Print and shaded views of the part. All mm, measured from the part's lowest x, y and z. A direction names the side the tool comes from. Coordinates: 2 decimals unless noted, no trailing zeros. Loops run counter-clockwise (first coordinate to the right, second up) from the corner with the lowest first, then second, coordinate; pieces in that order, holes last. Notation, with made-up numbers: M 44,30.5 L 59,30.5 A33 ccw 59,61.5 Z; hole C -24,62 d6. An arc over 180 degrees is marked long. Answer as a JSON object with one key per item and string values. Group by question number.
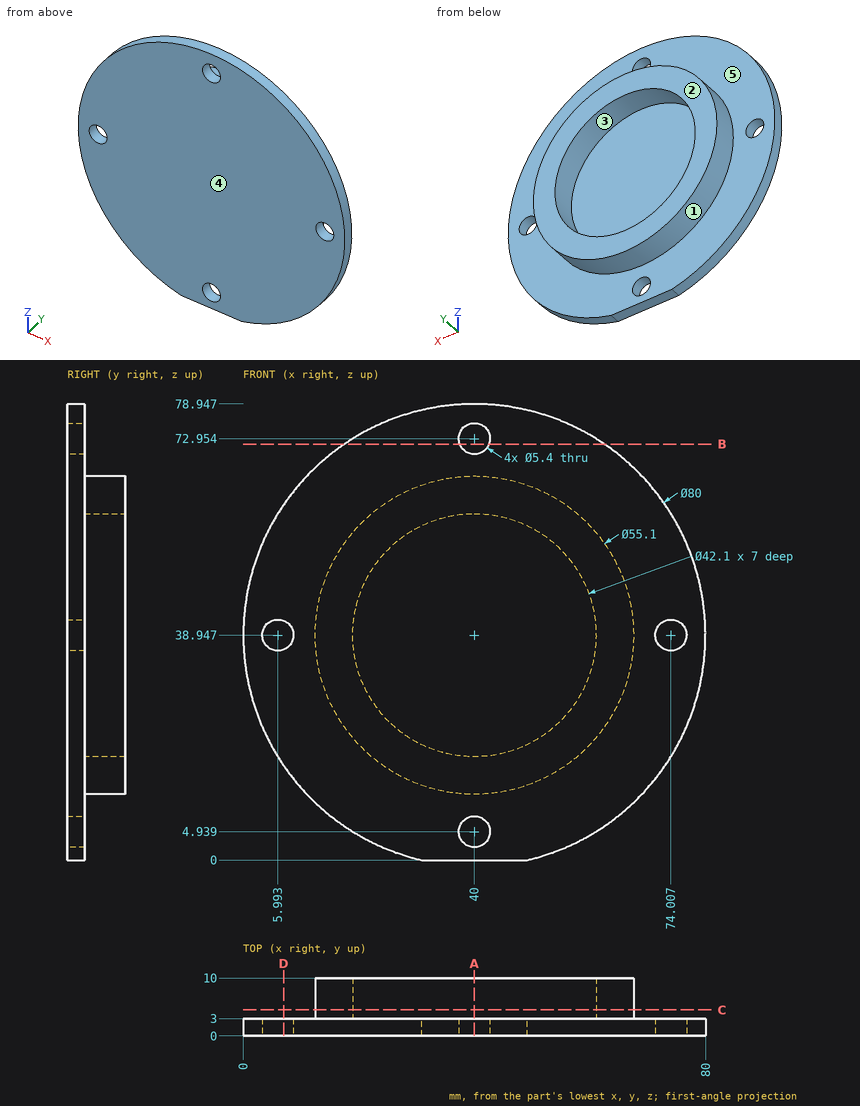
Item 1: Drill centre lines: L1, parallel to X at y = 5.25, z = 38; L2, parallel to Z at x = 55.5, y = 7.75 (1 decimal); L3, parallel to Z at x = 49, y = 8 (1 decimal). Where is each one in solid material? Low to high. Write a range as from..to.
Item 2: Slice it at D-D, the plane x = 7. Write the cut outline in (y, z).
Item 3: Slice it at C-C, the plane y = 4.5. Write the cut outline in (x, z).
Item 4: Tool access for the marked faces 4 and 5: list every direction of +Z, -Z, +X, -X, +Y, -Y with a clear straight run to the whole face (end or side of a thin tool).
Item 5: Pin check, flat tips, straight feed: pin 1 (6 mm diameter, centred on y = 7, z = 21.5, fed in from +X); pin 2 (8.5 mm diameter, centred on x = 40, z = 4.94, fed in from +Y); pin 3 (2 mm diameter, centred on y = 6.5, z = 12.5, fed in from +X) (1 decimal); pin 4 (2 mm diameter, centred on x = 45, z = 67, fed in from -Y). Stop position of each tip, or through.
Item 6: Slice it at B-B, the plane z = 72. Write the cut outline in (x, y) (1 decimal), then the cut area to 3 significant figures.
Item 7: Pull direction X, two halves, no side cores. Call the marked faces 1, 2 and 3: released by +X, released by -X, zero draft, split by the parting line, or undercut.
Item 8: Slice it at A-A, the plane x = 40. Write the cut outline in (y, z).
Computed:
{
 "1": {"L1": "12.47..18.97, 61.03..67.53", "L2": "16.2..24.7, 53.2..61.7", "L3": "12.9..19.9, 58..65"},
 "2": {"outline": "M 0,16.34 L 3,16.34 L 3,36.44 L 0,36.44 Z; M 0,41.45 L 3,41.45 L 3,61.55 L 0,61.55 Z"},
 "3": {"outline": "C 40,38.95 d55.1; hole C 40,38.95 d42.1"},
 "4": {"face 4": "+Z, -Z, +X, -X, -Y", "face 5": "+Y"},
 "5": {"pin 1": "x = 63.46", "pin 2": "y = 3", "pin 3": "x = 50.6", "pin 4": "y = 0"},
 "6": {"outline": "M 17.5,0 L 37.5,0 L 37.5,3 L 17.5,3 Z; M 42.5,0 L 62.5,0 L 62.5,3 L 42.5,3 Z", "area": "120 mm2"},
 "7": {"face 1": "split by the parting line", "face 2": "zero draft", "face 3": "undercut"},
 "8": {"outline": "M 0,0 L 3,0 L 3,2.24 L 0,2.24 Z; M 0,7.64 L 3,7.64 L 3,11.4 L 10,11.4 L 10,17.9 L 3,17.9 L 3,60 L 10,60 L 10,66.5 L 3,66.5 L 3,70.25 L 0,70.25 Z; M 0,75.65 L 3,75.65 L 3,78.95 L 0,78.95 Z"}
}
